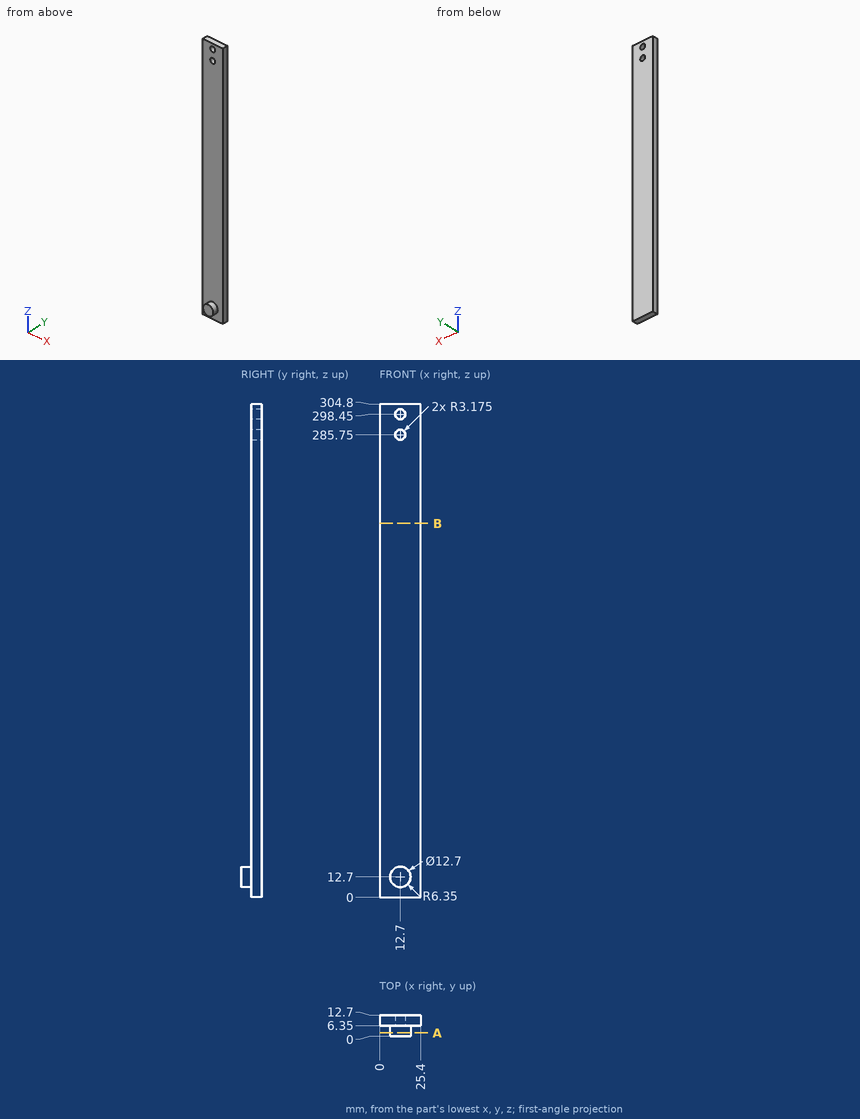
Check sheet for the drawn part. Datum: minimum x, y, z corner. Units: mm. Give positions to 0.01 mm unless a question says otherwise; leave off trailing zeros. Order: outer loops, then holes, each group sorted by start corner. A loop starts at its lowest first (then second) coordinate and runs counter-clockwise, first axis right, second up. Notation, with made-up numbers: (-20.5, 44) -> (14.5, 44) arc R8 cw to (14.5, 50) -> close; hole circle Ø11 at (-12.5, 0.25). An arc over 180 degrees is marked (long way). Return JSON: item names as keys, results as strings.
1. Cross-section at A-A, the plane y = 2. Record the cut outline in (x, z).
From the geometry:
{"outline": "circle Ø12.7 at (12.7, 12.7)"}
2. Go/stop test with flat-tipped pins: P1, Ø5, axis at y = 4.5, z = 170.5, coming from the +X side; P2, Ø1, axis at x = 16.5, y = 4, coming from the -Z side. Record where each tip stops, or that it passes through.
From the geometry:
{"P1": "x = 25.4", "P2": "z = 7.27"}
3. Cross-section at B-B, the plane z = 231. Record the cut outline in (x, y).
From the geometry:
{"outline": "(0, 6.35) -> (25.4, 6.35) -> (25.4, 12.7) -> (0, 12.7) -> close"}
4. Material ranges on probe 1 along Z at (x, y) = (11.5, 8); probe 2 along Z at (x, y) = (12, 7); probe 3 along Y at (x, z) = (17, 149), recorded low to high. Write a range as [from, to].
From the geometry:
{"probe 1": "[0, 282.81], [288.69, 295.51], [301.39, 304.8]", "probe 2": "[0, 282.65], [288.85, 295.35], [301.55, 304.8]", "probe 3": "[6.35, 12.7]"}
